from build123d import *

# Parameters (mm, degrees)
PAD_DEPTH            = 23
POCKET_DEPTH         = 25
SKETCH002_W          = 15
SKETCH002_H          = 3.5
PAD001_DEPTH         = 10
SKETCH003_W          = 3.5
SKETCH003_H          = 10
PAD002_DEPTH         = 40
SKETCH004_W          = 49.242171
SKETCH004_H          = 32.94012
PAD003_DEPTH         = 3
BODY_PLACEMENT_ANGLE = 90.375075


with BuildPart() as part:
    # Sketch → Pad (new body)
    with BuildSketch(Plane.YZ):
        with BuildLine():
            ThreePointArc((-10, 22.5), (-32.5, 0), (-10, -22.5))
            Line((-10, -22.5), (10, -22.5))
            ThreePointArc((10, -22.5), (32.5, 0), (10, 22.5))
            Line((-10, 22.5), (10, 22.5))
        make_face()
    extrude(amount=PAD_DEPTH)

    # Sketch001 (on Face6 of Pad) → Pocket (cut)
    with BuildSketch(Plane.YZ.offset(23)):
        with BuildLine():
            ThreePointArc((-9, 19), (-28, 0), (-9, -19))
            Line((-9, -19), (9, -19))
            ThreePointArc((9, -19), (28, 0), (9, 19))
            Line((-9, 19), (9, 19))
        make_face()
    extrude(amount=-POCKET_DEPTH, mode=Mode.SUBTRACT)

    # Sketch002 (on Face5 of Pocket) → Pad001 (join)
    with BuildSketch(Plane.YZ.offset(23)):
        with Locations((0, 20.75)):
            Rectangle(SKETCH002_W, SKETCH002_H)
    extrude(amount=PAD001_DEPTH)

    # Sketch003 (on Face13 of Pad001) → Pad002 (join)
    with BuildSketch(Plane.ZX.offset(7.5)):
        with Locations((20.75, 28)):
            Rectangle(SKETCH003_W, SKETCH003_H)
    extrude(amount=PAD002_DEPTH)

    # Sketch004 (on Face18 of Pad002) → Pad003 (join)
    with BuildSketch(Plane.ZX.offset(47.5)):
        with Locations((-2.121085, 16.52994)):
            Rectangle(SKETCH004_W, SKETCH004_H)
    extrude(amount=PAD003_DEPTH)


with BuildPart() as part_1:
    # Body placement: moved
    add(part.part.moved(Location((0, 0.13901, -0.480614))).rotate(Axis((0, 0.13901, -0.480614), (-1, 0, 0)), BODY_PLACEMENT_ANGLE))


solid = part_1.part
Verification items for the finished model (mm, model axes). A direction names the side the tool comes from. Give positions to 0.01 mm unless a question says otherwise; leave off trailing zeros. Loops run counter-clockwise (first coordinate to the right, second up) from the corner with the lowest first, then second, coordinate; pieces in that order, holes last.
1) Sectioned sample at C-C, the plane z = -16.5. Enter the section's corners in (x, y), then the cut area to 3 significant figures.
2) Depth check by flat-ended pin: pin 1 Ø3 at (y, z) = (21.5, -28.5) entering from -X; pin 2 Ø10 at (x, y) = (19.5, -14) entering from -Z; pin 3 Ø1 at (x, z) = (17.5, -29) entering from +Y. Enter the tip coordinate at first touch or a pass-through.
3) Sectioned sample at A-A, the plane z = -27. Enter the section's corners in (x, y).
4) Thickness scan on line 1 along Z through (x, y) = (11, 3.5); line 2 along Z through (x, y) = (3.5, -13); line 3 along Y through (x, z) = (18, 6.5). Record the ranges inside material, lowest first.
5) Sectioned sample at D-D, the plane x = 3.5. Enter the section's corners in (y, z).
6) Sectioned sample at B-B, the plane y = -15. Enter the section's corners in (x, z), then the cut area to 3 significant figures.
7) Set-up check for faces 1 (the flat face through (23, 21, -33)), 2 (the cylindrical face through (11.66, 0.74, 27.51)), 3 (the flat face through (0, -20, 0)), 4 (the flat face through (23, -20, 2)): record each of +Z, -Z, +X, -X, +Y, -Y from which the full face is reachable in a straight line by a thin tool's end or side.
8) Draft check along Z on faces 5 (the cylindrical face through (11.34, -0.57, -32.97)), 6 (the flat face through (33, 20, -31)). Enter one of: pulls with the +Z half, pulls with the -Z half, needs draft (parallel to the pull), parting line crosses it, or undercut.
Answers:
1. outline: (0, -21.61) - (23, -21.61) - (23, -17.58) - (0, -17.58) - close; (0, 17.74) - (23, 17.74) - (23, 19.03) - (33, 19.03) - (33, 22.53) - (23, 22.53) - (23, 21.75) - (0, 21.75) - close
1. area: 220 mm2
2. pin 1: stops at x = 23
2. pin 2: stops at z = -50.92
2. pin 3: stops at y = 13.55
3. outline: (0, -15.2) - (23, -15.2) - (23, -7.27) - (0, -7.27) - close; (0, 7.43) - (23, 7.43) - (23, 15.35) - (0, 15.35) - close; (23, 18.97) - (33, 18.97) - (33, 22.47) - (23, 22.47) - close
4. line 1: z = -51 to -48, -32.72 to -28.17, 27.23 to 31.78
4. line 2: z = -50.9 to -47.9, -28.79 to -23.26, 22.19 to 27.74
4. line 3: y = -22.32 to -18.82, 19.19 to 22.69
5. outline: (-26.93, -50.8) - (22.31, -51.13) - (22.33, -48.13) - (-26.91, -47.8) - close; (-22.43, -10.33) arc R22.5 ccw to (22.57, -10.63) - (22.7, 9.37) arc R22.5 ccw to (-22.3, 9.67) - close; hole (-18.92, -9.36) arc R19 ccw to (19.08, -9.6) - (19.2, 8.39) arc R19 ccw to (-18.8, 8.64) - close
6. outline: (0, -27.18) - (23, -27.18) - (23, -21.04) - (0, -21.04) - close; (0, 19.92) - (23, 19.92) - (23, 26.1) - (0, 26.1) - close; (0.06, -50.88) - (33, -50.88) - (33, -47.88) - (0.06, -47.88) - close
6. area: 382 mm2
7. face 1: -X, +Y
7. face 2: +X, -X
7. face 3: +Z, -Z, -X, +Y, -Y
7. face 4: +Z, +X, -Y
8. face 5: undercut
8. face 6: needs draft
